Check sheet for the modelled part. Datum: model origin and axes. Units: mm. A direction names the side the tool comes from. Round coordinates to 2 decimals unless told otherwise and drop trailing zeros. Order: outer loops, then holes, each group sorted by start corner. A loop starts at its lowest first (then second) coordinate and runs counter-clockwise, first axis right, second up.
(1) Sectioned sample at B-B, the plane x = 68.5. Enter the section's corners in (y, z), and give its area (3 significant figures).
(2) Depth check by flat-ended pin: pin 1 (10 mm diameter, centred on x = 14, y = -2, fed in from -Z); pin 2 (5 mm diameter, centred on x = 56, z = 5.5, fed in from +Y); pin 3 (3 mm diameter, centred on x = 81.5, y = 0, fed in from +Z); pin 4 (2.5 mm diameter, centred on x = -9.83, y = 0.28, fed in from -Z). Enter the tip coordinate at first touch or a pass-through.
(3) Mould release check, pull along Y, two halves, no side actions. Record for faces 1 (the cylindrical face through (132.751, -11.463, 2.601)), 2 (the flat face through (54, 0, 0)), 3 (the flat face through (125.32, -0.24, 1.93)): released by +Y, released by -Y, zero draft, split by the parting line, or undercut.
(4) Tool access check on faces 4 (the flat face through (55, -4.724, 2)), 5 (the flat face through (124, -1, -3)). Record the directions out of +Z, -Z, +X, -X, +Y, -Y that give a thin tool (end or side, any length) a straight path to the whole face; none if there is none.
(5) Thickness scan on probe 1 along Y at (x, z) = (57, 1); probe 2 along Z at (x, y) = (4, 1); probe 3 along Y at (x, z) = (-8.5, 3). Record the ranges inside material, lowest first.
(6) Sectioned sample at A-A, the plane z = -1.5. Enter the section's corners in (x, y) (3 decimals), and give its area (3 significant figures).
```python
from build123d import *

# Parameters (mm, degrees)
SKETCH_1_R      = 2.1
EXTRUDE_1_DEPTH = 4
FILLET_1_R      = 2
SKETCH_2_R      = 2
EXTRUDE_2_DEPTH = 3


with BuildPart() as part:
    # 草图1 → 凸台-拉伸1 (new body)
    with BuildSketch(Plane.XY):
        Polygon((125.165745856, -4.723756906), (116.774749545, 5.276243094), (-14.834254144, 5.276243094), (-14.834254144, -4.723756906), align=None)
        with Locations((-9.834254144, 0.276243094)):
            Circle(SKETCH_1_R, mode=Mode.SUBTRACT)
    extrude(amount=EXTRUDE_1_DEPTH)

    # 圆角1
    fillet_1_edges = [part.edges().sort_by_distance(p)[0] for p in [
        (-14.834254144, 5.276243094, 2),
        (-14.834254144, -4.723756906, 2),
    ]]
    fillet(fillet_1_edges, radius=FILLET_1_R)

    # 草图2 → 凸台-拉伸2 (add)
    with BuildSketch(Plane(origin=(71.124278553, 59.680355902, 0), x_dir=(0, 0, -1), z_dir=(0.7660444431189745, 0.6427876096865437, 0))):
        Polygon((-4, -61.019525429), (3, -61.019525429), (3, -101.019525429), (-7, -101.019525429), (-7, -61.019525429), align=None)
        with Locations(Location((-2, -66.019525429, 0), (0, 0, 90))):
            Circle(SKETCH_2_R, mode=Mode.SUBTRACT)
        with Locations(Location((-2, -96.019525429, 0), (0, 0, 90))):
            Circle(SKETCH_2_R, mode=Mode.SUBTRACT)
    extrude(amount=EXTRUDE_2_DEPTH)


solid = part.part
```
Derived:
1. outline: (-4.72, 0) - (5.28, 0) - (5.28, 4) - (-4.72, 4) - close
1. area: 40.0 mm2
2. pin 1: stops at z = 0
2. pin 2: stops at y = 5.28
2. pin 3: stops at z = 4
2. pin 4: passes through
3. face 1: undercut
3. face 2: zero draft
3. face 3: released by +Y
4. face 4: +Z, -Z, -X, -Y
4. face 5: -Z, +X, -X, +Y, -Y
5. probe 1: y = -4.72 to 5.28
5. probe 2: z = 0 to 4
5. probe 3: y = -4.72 to -1.35, 1.9 to 5.28
6. outline: (110.347, 12.937) - (136.058, -17.705) - (138.357, -15.777) - (112.645, 14.865) - close
6. area: 120 mm2
